Check sheet for the modelled part. Datum: model origin and axes. Units: mm. A direction names the side the tool comes from. Coordinates: 2 decimals unless noted, no trailing zeros. Order: outer loops, then holes, each group sorted by start corner. A loop starts at its lowest first (then second) coordinate and runs counter-clockwise, first axis right, second up. Notation, with made-up numbers: M 10.5,19 L 37.5,19 A21 cw 37.5,32 Z; hole C 14.5,46.25 d2. An arc over 180 degrees is marked long. Answer in a Markdown table with one row per item. Add a question column.
from build123d import *

# Parameters (mm, degrees)
F1_W            = 42
F1_H            = 42
F2_DEPTH        = 40
F3_R            = 11
F4_DEPTH        = 2
F5_R            = 2.5
F6_DEPTH        = 21
F8_D            = 4.5
F8_COPIES_COUNT = 4
F9_SIZE         = 4


# Not quite as in the source:
# - a pattern or mirror of a feature is missing from the dataset's text; its kind, count and spacing are read off the source's solid


with BuildPart() as f2:
    # F1 (on Top) → F2 (new body)
    with BuildSketch(Plane.XY):
        Rectangle(F1_W, F1_H)
    extrude(amount=F2_DEPTH)

    # F3 (on face) → F4 (join)
    with BuildSketch(Plane.XY.offset(40)):
        Circle(F3_R)
    extrude(amount=F4_DEPTH)

    # F5 (on face) → F6 (join)
    with BuildSketch(Plane.XY.offset(42)):
        Circle(F5_R)
    extrude(amount=F6_DEPTH)

    # F8 (through all)
    with Locations(Plane.XY.offset(40)):
        with Locations((15.5, 15.5)):
            f8 = Hole(F8_D / 2)

    # F8_copies: F8 ×4 about axis
    f8_copies_axis = Axis((0, 0, 0), (0, 0, 1))
    for i in range(1, F8_COPIES_COUNT):
        add(f8.rotate(f8_copies_axis, i * 360 / F8_COPIES_COUNT), mode=Mode.SUBTRACT)

    # F9
    f9_edges = [f2.edges().sort_by_distance(p)[0] for p in [
        (21, 21, 20),
        (21, -21, 20),
        (-21, -21, 20),
        (-21, 21, 20),
    ]]
    chamfer(f9_edges, length=F9_SIZE)


solid = f2.part
1. Section check A-A on x = 15.5. Enter the section's corners in (y, z), then the cut area to 3 significant figures.
2. Release check for a two-part mould opening along Y. For faces 3 (the flat face through (0, 0, 63)), 4 (the cylindrical face through (-14.462, -13.504, 19.72)), 5 (the cylindrical face through (-2.38, -10.74, 40.99)) record: released by +Y, released by -Y, zero draft, split by the parting line, or undercut.
3. Section check C-C on x = 0. Enter the section's corners in (y, z), then the cut area to 3 significant figures.
4. Set-up check for faces 1 (the cylindrical face through (-0.54, -2.44, 52.35)), 2 (the flat face through (0, 21, 20)): record each of +Z, -Z, +X, -X, +Y, -Y from which the full face is reachable in a straight line by a thin tool's end or side.
5. Go/stop test with flat-tipped pins: pin 1 Ø4 at (x, y) = (15.5, 15.5) entering from -Z; pin 2 Ø6 at (x, y) = (15.5, -15.5) entering from +Z. Record where each tip stops, or that it passes through.
6. Section check D-D on z = 7. Enter the section's corners in (x, y), then the cut area to 3 significant figures.
7. Scan lines: line 1 (X direction, y = -14, z = 17.5); line 2 (Y direction, x = 15, z = 14). Record each from-to range of solid material in increasing order.
Result sheet:
| question | item | result |
|---|---|---|
| 1 | outline | M -21,0 L -17.75,0 L -17.75,40 L -21,40 Z; M -13.25,0 L 13.25,0 L 13.25,40 L -13.25,40 Z; M 17.75,0 L 21,0 L 21,40 L 17.75,40 Z |
| 1 | area | 1,320 mm^2 |
| 2 | face 3 | zero draft |
| 2 | face 4 | undercut |
| 2 | face 5 | split by the parting line |
| 3 | outline | M -21,0 L 21,0 L 21,40 L 11,40 L 11,42 L 2.5,42 L 2.5,63 L -2.5,63 L -2.5,42 L -11,42 L -11,40 L -21,40 Z |
| 3 | area | 1,830 mm^2 |
| 4 | face 1 | +Z |
| 4 | face 2 | +Z, -Z, +X, -X, +Y |
| 5 | pin 1 | through |
| 5 | pin 2 | z = 40 |
| 6 | outline | M -21,-17 L -17,-21 L 17,-21 L 21,-17 L 21,17 L 17,21 L -17,21 L -21,17 Z; hole C -15.5,-15.5 d4.5; hole C -15.5,15.5 d4.5; hole C 15.5,-15.5 d4.5; hole C 15.5,15.5 d4.5 |
| 6 | area | 1,670 mm^2 |
| 7 | line 1 | -21 to -17.18, -13.82 to 13.82, 17.18 to 21 |
| 7 | line 2 | -21 to -17.69, -13.31 to 13.31, 17.69 to 21 |
